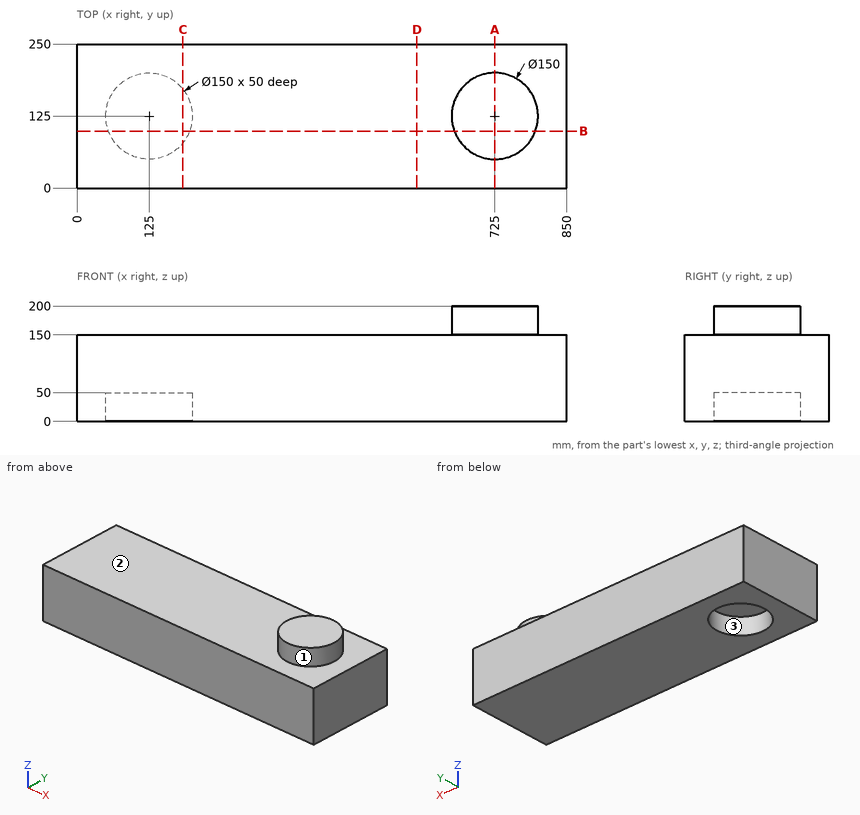
Source: three-view drawing plus pictorial views. Frame: mm from the lowest corner of the part. Give positions to 0.01 mm unless a question says otherwise; leave off trailing zeros. Loops run counter-clockwise (first coordinate to the right, second up) from the corner with the lowest first, then second, coordinate; pieces in that order, holes last. Notation, with made-up numbers: (66, 87) -> (101, 87) arc R17 cw to (101, 109) -> close; hole circle Ø8 at (78.25, -26.75). An arc over 180 degrees is marked (long way). Put each result on its own line as item: value. Start each with the question number.
1) Draft query along Y for the marked faces 1, 2 and 3. Return one class per face: released by +Y, released by -Y, zero draft, split by the parting line, or undercut.
2) Cut plane B-B (y = 99). Return loops of the section in (x, z).
3) Cut plane D-D (x = 589.5). Return loops of the section in (y, z).
4) Cut plane A-A (x = 725). Return loops of the section in (y, z).
5) Material intervals for probe 1 along Y at (x, z) = (125, 30.5); probe 2 along Z at (x, y) = (583, 164.5); probe 3 along Y at (x, z) = (154.5, 31), sorted ascending.
6) Cut plane C-C (x = 183.5). Return loops of the section in (y, z).
7) Contact query for a flat-ended pin moving along its axis: P1, Ø2, axis at x = 492.5, y = 158, coming from the +Z side. Output: stop coordinate, or through.
Results are:
1. face 1: split by the parting line
1. face 2: zero draft
1. face 3: undercut
2. outline: (0, 0) -> (54.65, 0) -> (54.65, 50) -> (195.35, 50) -> (195.35, 0) -> (850, 0) -> (850, 150) -> (795.35, 150) -> (795.35, 200) -> (654.65, 200) -> (654.65, 150) -> (0, 150) -> close
3. outline: (0, 0) -> (250, 0) -> (250, 150) -> (0, 150) -> close
4. outline: (0, 0) -> (250, 0) -> (250, 150) -> (200, 150) -> (200, 200) -> (50, 200) -> (50, 150) -> (0, 150) -> close
5. probe 1: y = 0 to 50, 200 to 250
5. probe 2: z = 0 to 150
5. probe 3: y = 0 to 56.05, 193.95 to 250
6. outline: (0, 0) -> (78.07, 0) -> (78.07, 50) -> (171.93, 50) -> (171.93, 0) -> (250, 0) -> (250, 150) -> (0, 150) -> close
7. P1: stops at z = 150
